The figure shows three views and two pictorial views of one solid part (mm, origin at its lowest corner). Answer the questions. Give positions to 0.01 mm unless a question says otherwise; leave off trailing zeros. Loops run counter-clockwise (first coordinate to the right, second up) from the corner with the lowest first, then second, coordinate; pieces in that order, holes last.
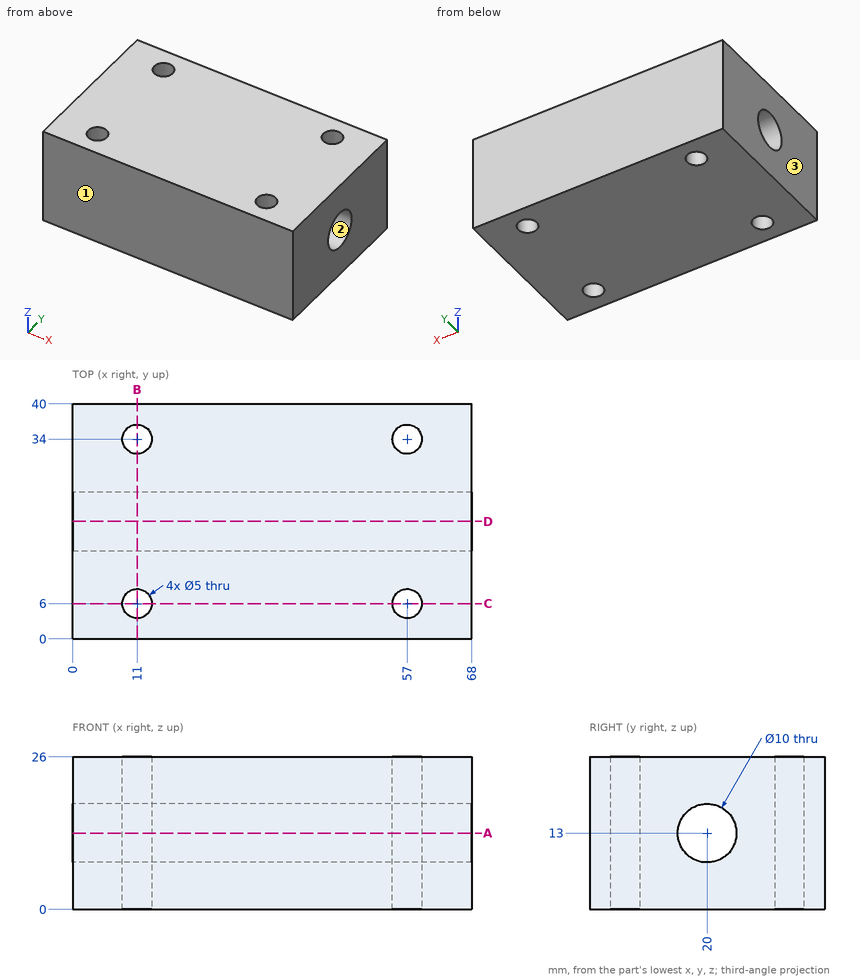
Q1. Section D-D on y = 20 is taken. Give the vertices of the cut face in (x, z), plus the area to 3 significant figures.
Q2. Determine the mould class of the marked faces 1, 2 and 3 for opening direction Y: +Y half, -Y half, draft (parallel to the pull), parting line (faces both ways), or undercut.
Q3. Given pin 1 (4.5 mm diameter, centred on x = 57, y = 6, fed in from -Z), flat-ended and moving along its own axis, determine where the tip first touches the part or whether it passes through.
Q4. Section A-A on z = 13 is taken. Give the vertices of the cut face in (x, y).
Q5. Section B-B on x = 11 is taken. Give the vertices of the cut face in (y, z), plus the area to 3 significant figures.
Q6. Consider line 1 along Y through (x, z) = (9, 7); line 2 along Z through (x, y) = (30, 20); line 3 along Y through (x, z) = (40.5, 9.75). Determine where each line is inside the solid, lowest interval first.
Q7. Section C-C on y = 6 is taken. Give the vertices of the cut face in (x, z).
Check result:
1. outline: (0, 0) - (68, 0) - (68, 8) - (0, 8) - close; (0, 18) - (68, 18) - (68, 26) - (0, 26) - close
1. area: 1,090 mm2
2. face 1: -Y half
2. face 2: undercut
2. face 3: draft
3. pin 1: passes through
4. outline: (0, 0) - (68, 0) - (68, 15) - (0, 15) - close; (0, 25) - (68, 25) - (68, 40) - (0, 40) - close; hole circle Ø5 at (11, 6); hole circle Ø5 at (11, 34); hole circle Ø5 at (57, 6); hole circle Ø5 at (57, 34)
5. outline: (0, 0) - (3.5, 0) - (3.5, 26) - (0, 26) - close; (8.5, 0) - (31.5, 0) - (31.5, 26) - (8.5, 26) - close; (36.5, 0) - (40, 0) - (40, 26) - (36.5, 26) - close; hole circle Ø10 at (20, 13)
5. area: 701 mm2
6. line 1: y = 0 to 4.5, 7.5 to 32.5, 35.5 to 40
6. line 2: z = 0 to 8, 18 to 26
6. line 3: y = 0 to 16.2, 23.8 to 40
7. outline: (0, 0) - (8.5, 0) - (8.5, 26) - (0, 26) - close; (13.5, 0) - (54.5, 0) - (54.5, 26) - (13.5, 26) - close; (59.5, 0) - (68, 0) - (68, 26) - (59.5, 26) - close
